For this review, take the finished solid that the model builds, in its own axes (mm). Face numbers are marked on the shaded views. A direction names the side the tool comes from. Round coordinates to 2 decimals unless told otherwise and drop trailing zeros. Loops run counter-clockwise (first coordinate to the right, second up) from the corner with the lowest first, then second, coordinate; pieces in that order, holes last.
1. Clearance check with flat-ended pins moving along their axes: pin 1 Ø1.1 at (y, z) = (22.5, 0.5) entering from +X; pin 2 Ø1.9 at (x, z) = (-50.5, 2.5) entering from -Y; pin 3 Ø2 at (x, z) = (-51.5, 0.5) entering from +Y. State where each tip first meets the part, or that it passes through.
2. To check wall thickness, follow line 1 along Y through (x, z) = (-50.3, 4.2); line 2 along Y through (x, z) = (-48.7, 2.55); line 3 along Z through (x, y) = (-50.1, 26). State the ranges of each line that lie inside material, in increasing order.
3. Consider section D-D on z = 1.4. State the section outline as (x, y) points.
4. Consider section B-B on y = 30. State the section outline as (x, z) points.
5. Tool access review of the marked faces 1 and 2: name each direction out of +Z, -Z, +X, -X, +Y, -Y from which nothing blocks a thin tool from reaching the whole face with its end or side.
6. Consider section A-A on z = 2.95. State the section outline as (x, y) points, then the cut area to 3 significant figures.
7. Consider section C-C on x = -50.25. State the section outline as (y, z) points, then the cut area to 3 significant figures.
from build123d import *

# Parameters (mm, degrees)
F0_W     = 1.8106922507
F0_H     = 10.411484167
F1_DEPTH = 1.016
F3_DEPTH = 10.16
F4_R     = 1.3504663761
F5_DEPTH = 25.4


with BuildPart() as f1:
    # F0 (on Top) → F1 (new body)
    with BuildSketch(Plane.XY):
        with Locations((-50.0065051019, 23.5388400033)):
            Rectangle(F0_W, F0_H)
    extrude(amount=F1_DEPTH)

    # F2 (on face) → F3 (join)
    with BuildSketch(Plane(origin=(0, 28.7445820868, 0), x_dir=(-1, 0, 0), z_dir=(0, 1, 0))):
        with BuildLine():
            ThreePointArc((50.9118512273, 0.6882785491), (51.6883442883, 1.4132903762), (51.9750051019, 2.4362318218))
            ThreePointArc((51.9750051019, 2.4362318218), (48.9835636563, 4.1180710082), (49.1011589766, 0.6882785491))
            Line((49.1011589766, 0.6882785491), (49.1011589766, 1.016))
            Line((49.1011589766, 1.016), (50.9118512273, 1.016))
            Line((50.9118512273, 1.016), (50.9118512273, 0.6882785491))
        make_face()
    extrude(amount=-F3_DEPTH)

    # F4 (on face) → F5 (join)
    with BuildSketch(Plane(origin=(0, 28.7445820868, 0), x_dir=(-1, 0, 0), z_dir=(0, 1, 0))):
        with Locations((50.0065051019, 2.4362318218)):
            Circle(F4_R)
    extrude(amount=F5_DEPTH)


solid = f1.part
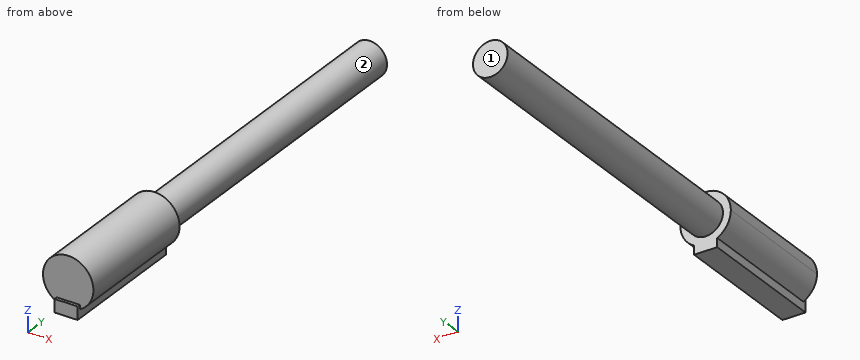
Resolved:
1. pin 1: stops at x = -48.61
1. pin 2: stops at y = 18.58
1. pin 3: stops at y = 28.74
2. line 1: y = 18.58 to 28.74
2. line 2: y = 18.58 to 54.14
2. line 3: z = 0 to 4.4
3. outline: (-51.68, 18.58) - (-48.33, 18.58) - (-48.33, 28.74) - (-49.14, 28.74) - (-49.14, 54.14) - (-50.87, 54.14) - (-50.87, 28.74) - (-51.68, 28.74) - close
4. outline: circle Ø2.7 at (-50.01, 2.44)
5. face 1: +Z, -Z, +X, -X, +Y
5. face 2: +Y
6. outline: (-51.91, 18.58) - (-48.11, 18.58) - (-48.11, 28.74) - (-48.76, 28.74) - (-48.76, 54.14) - (-51.26, 54.14) - (-51.26, 28.74) - (-51.91, 28.74) - close
6. area: 102 mm2
7. outline: (18.33, 0) - (28.74, 0) - (28.74, 1.11) - (54.14, 1.11) - (54.14, 3.76) - (28.74, 3.76) - (28.74, 4.39) - (18.58, 4.39) - (18.58, 1.02) - (18.33, 1.02) - close
7. area: 112 mm2
